Model file for the job. Use its own axes, mm. Face numbers are marked on the shaded views. Round coordinates to 2 decimals unless told otherwise and drop trailing zeros. Order: outer loops, then holes, each group sorted by start corner. A loop starts at its lowest first (then second) coordinate and runs counter-clockwise, first axis right, second up. Notation, with made-up numbers: M 5,26.25 L 12,26.25 A33 cw 12,62.25 Z; hole C 59.5,19 d8. An arc over 180 degrees is marked long. Return JSON: item names as keys, results as strings. Group by question number.
Item 1: Slice it at A-A on x = -0.5. Write the cut outline in (y, z).
Item 2: Probe line 1 along X through (y, z) = (-1.8, 0.5); line 2 along Z through (x, y) = (0.75, -1.75); line 3 along Y through (x, z) = (-1, 0.95). List the from-to ranges inside material, lowest first.
Item 3: Slice it at B-B on z = 0.4. Write the cut outline in (x, y).
Item 4: Pull direction Z, two halves, no side cores. Call the marked faces 1, 2 and 3: pulls with the +Z half, pulls with the -Z half, needs draft (parallel to the pull), parting line crosses it, or undercut.
from build123d import *

# Parameters (mm, degrees)
SKETCH2_W           = 7
SKETCH2_H           = 5
BOSS_EXTRUDE1_DEPTH = 2
SKETCH3_W           = 6.5
SKETCH3_H           = 1.5
CUT_EXTRUDE1_DEPTH  = 0.5


with BuildPart() as part:
    # Sketch2 → Boss-Extrude1 (new body)
    with BuildSketch(Plane.XY):
        with Locations((0, 0.3508563)):
            Rectangle(SKETCH2_W, SKETCH2_H)
    extrude(amount=BOSS_EXTRUDE1_DEPTH)

    # Sketch3 → Cut-Extrude1 (cut)
    with BuildSketch(Plane.XZ.offset(2.1491437)):
        with Locations((0, 1)):
            Rectangle(SKETCH3_W, SKETCH3_H)
    extrude(amount=-CUT_EXTRUDE1_DEPTH, mode=Mode.SUBTRACT)


solid = part.part
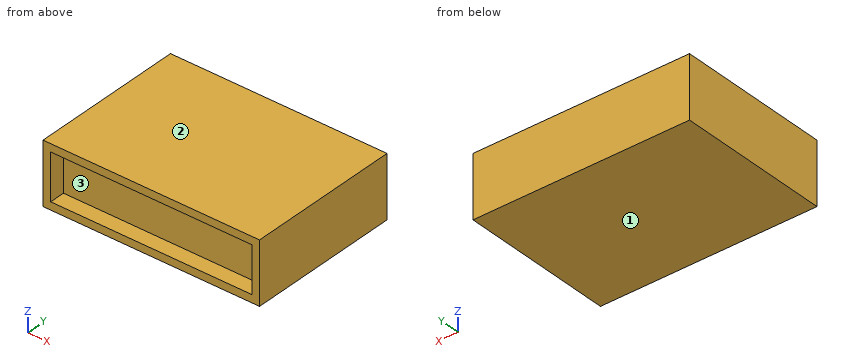
Output values:
{
 "1": {"outline": "M -2.15,0 L 2.85,0 L 2.85,2 L -2.15,2 L -2.15,1.75 L -1.65,1.75 L -1.65,0.25 L -2.15,0.25 Z"},
 "2": {"line 1": "-3.5 to -3.25, 3.25 to 3.5", "line 2": "0 to 0.25, 1.75 to 2", "line 3": "-1.65 to 2.85"},
 "3": {"outline": "M -3.5,-2.15 L -3.25,-2.15 L -3.25,-1.65 L 3.25,-1.65 L 3.25,-2.15 L 3.5,-2.15 L 3.5,2.85 L -3.5,2.85 Z"},
 "4": {"face 1": "pulls with the -Z half", "face 2": "pulls with the +Z half", "face 3": "undercut"}
}
